Can you work these out from the model? Positions are in its coordinate system, mm. A direction names the side the tool comes from. Round coordinates to 2 decimals unless told otherwise and drop trailing zeros. Loops run counter-clockwise (first coordinate to the right, second up) from the corner with the lowest first, then second, coordinate; pieces in that order, holes last. Notation, with made-up numbers: (60, 63.25) -> (89, 63.25) arc R14 cw to (89, 67.25) -> close; hole circle Ø2 at (66, -8.5). An arc over 180 degrees is marked (long way). Write each question's results on one line, items separated by ' | '.
from build123d import *

# Parameters (mm, degrees)
SKETCH1_R           = 3.175
SKETCH1_R_2         = 1.5875
BOSS_EXTRUDE1_DEPTH = 9.525
BOSS_EXTRUDE2_DEPTH = 19.05
SKETCH4_R           = 1.5875
CUT_EXTRUDE1_DEPTH  = 20.0500001
CUT_EXTRUDE2_START  = -3.175
SKETCH5_R           = 3.175
SKETCH5_R_2         = 2.38125
CUT_EXTRUDE2_DEPTH  = 4.7625


with BuildPart() as part:
    # Sketch1 → Boss-Extrude1 (new body)
    with BuildSketch(Plane.XY):
        Circle(SKETCH1_R)
        Circle(SKETCH1_R_2, mode=Mode.SUBTRACT)
    extrude(amount=BOSS_EXTRUDE1_DEPTH)

    # Sketch3 → Boss-Extrude2 (add)
    with BuildSketch(Plane.ZY.offset(9.525)):
        with BuildLine():
            Line((-1.085913955, -2.983524071), (-0.542956978, -1.491762035))
            ThreePointArc((-0.542956978, -1.491762035), (1.5875, 0), (-0.542956978, 1.491762035))
            Line((-0.542956978, 1.491762035), (-1.085913955, 2.983524071))
            ThreePointArc((-1.085913955, 2.983524071), (3.175, 0), (-1.085913955, -2.983524071))
        make_face()
    extrude(amount=-BOSS_EXTRUDE2_DEPTH)

    # Sketch4 → Cut-Extrude1 (cut, through all)
    with BuildSketch(Plane.ZY.offset(9.525)):
        Circle(SKETCH4_R)
    extrude(amount=-CUT_EXTRUDE1_DEPTH, mode=Mode.SUBTRACT)

    # Sketch5 → Cut-Extrude2 (cut)
    with BuildSketch(Plane(origin=(0, 0, 0), x_dir=(0, 0, -1), z_dir=(1, 0, 0)).offset(CUT_EXTRUDE2_START)):
        Circle(SKETCH5_R)
        Circle(SKETCH5_R_2, mode=Mode.SUBTRACT)
    cut_extrude2 = extrude(amount=-CUT_EXTRUDE2_DEPTH, mode=Mode.SUBTRACT)

    # Mirror1: Cut-Extrude2 across plane
    add(cut_extrude2.mirror(Plane(origin=(0, 0, 0), x_dir=(0, 0, 1), z_dir=(1, 0, 0))), mode=Mode.SUBTRACT)


solid = part.part
1. Will these pins go through, and if not, where does the flat tip stop? pin 1 (1 mm diameter, centred on x = 3.5, z = 1, fed in from -Y); pin 2 (3 mm diameter, centred on x = 0, y = 0, fed in from +Z) (3 decimals); pin 3 (1 mm diameter, centred on x = 1.5, z = 1, fed in from +Y).
Final values:
pin 1: y = -3.11 | pin 2: z = 3.175 | pin 3: y = 3.14
2. We'd pull the mould along X, two halves only. Please class faces 5 (the face through (-8.742, 0.085, 3.174)), 6 (the face through (-9.525, 1, 2)), 7 (the face through (-3.17, 0.14, 5.75)), 8 (the face through (-0.022, 0.023, 3.175)): pulls with the +X half, pulls with the -X half, needs draft (parallel to the pull), parting line crosses it, or undercut.
Final values:
face 5: needs draft | face 6: pulls with the -X half | face 7: parting line crosses it | face 8: undercut
3. Please list where these lines run through material, in increasing order: line 1 (X direction, y = -1.75, z = 2.5) (1 decimal); line 2 (Y direction, x = 0, z = 7.5) (1 decimal). Write a range as from..to.
Final values:
line 1: -9.5..-7.9, -3.2..3.2, 7.9..9.5 | line 2: -3.2..-1.6, 1.6..3.2
4. On a 3-axis mill with a long thin cutter (end or side, diameter ignored), from which of +Z, -Z, +X, -X, +Y, -Y can I reach the whole of each face in a straight line? I mean faces 1 (the face through (8.72, 0.085, 3.174)), 2 (the face through (5.52, 0.06, 2.38)), 3 (the face through (0.661, -3.175, -0.05)), 4 (the face through (-0.75, 3.172, -0.135)). Say none if no direction works.
Final values:
face 1: +X | face 2: none | face 3: -Y | face 4: +Y
5. If we section it at D-D (x = -7): List the corners of the cut face in (y, z) for me (1 decimal), then the cut area to 3 significant figures.
Final values:
outline: (-2.2, -0.8) -> (-1.5, -0.5) arc R1.6 cw (long way) to (1.5, -0.5) -> (2.2, -0.8) arc R2.4 ccw (long way) to start | area: 6.05 mm2
